from build123d import *

# Parameters (mm, degrees)
BOSS_EXTRUDE1_DEPTH = 152.4
SKETCH2_R           = 9.525
CUT_EXTRUDE1_DEPTH  = 187.6511184
CIRPATTERN1_COUNT   = 9
CIRPATTERN1_ANGLE   = 240


with BuildPart() as part:
    # Sketch1 → Boss-Extrude1 (new body)
    with BuildSketch(Plane.XY):
        with BuildLine():
            Line((0, 76.2), (0, 0))
            Line((0, 0), (76.2, 0))
            ThreePointArc((76.2, 0), (-53.881536726, -53.881536726), (0, 76.2))
        make_face()
    extrude(amount=-BOSS_EXTRUDE1_DEPTH)

    # Sketch2 → Cut-Extrude1 (cut, through all)
    with BuildSketch(Plane.XY):
        with Locations((-13.969757959, 52.135846474)):
            Circle(SKETCH2_R)
    cut_extrude1 = extrude(amount=-CUT_EXTRUDE1_DEPTH, mode=Mode.SUBTRACT)

    # CirPattern1: Cut-Extrude1 ×9 about axis, 1 skipped
    cirpattern1_axis = Axis((0, 0, 0), (0, 0, 1))
    add([cut_extrude1.rotate(cirpattern1_axis, i * CIRPATTERN1_ANGLE / (CIRPATTERN1_COUNT - 1)) for i in range(1, CIRPATTERN1_COUNT) if i not in (3,)], mode=Mode.SUBTRACT)


solid = part.part
The listing builds one solid part. Answer for the finished solid, in the listing's coordinates (mm). A direction names the side the tool comes from. Round coordinates to 2 decimals unless told otherwise and drop trailing zeros. Order: outer loops, then holes, each group sorted by start corner. A loop starts at its lowest first (then second) coordinate and runs counter-clockwise, first axis right, second up. Notation, with made-up numbers: M -31,77.25 L 11,77.25 A18 ccw 11,83.25 Z; hole C -19,2 d1. An arc over 180 degrees is marked long. Answer in a Markdown table with one row per item. Add a question column.
1) Which of the six approach directions +Z, -Z, +X, -X, +Y, -Y give full straight-line access (tool end or side, diameter ignored) to faces 5 (the face through (-16, -16, -152.4)), 6 (the face through (0, 39, -75))?
2) Flat-ended cylindrical pins translate along their axes: pin 1 Ø12 at (y, z) = (23, -68) entering from -X; pin 2 Ø1 at (x, y) = (46, -48.5) entering from +Z; pin 3 Ø2 at (x, z) = (2.5, -24) entering from +Y; pin 4 Ø12 at (y, z) = (-22.5, -134) entering from -X. Find the tip coordinate at first contact, or state that the pin passes through.
3) The part is cut by section C-C on z = -35. Count the separate pieces of the cut face and the enclosed holes in it, plus the area to 3 significant figures.
4) Consider line 1 along X through (y, z) = (-49, -89); line 2 along Y through (x, z) = (-37.5, -88); line 3 along Y through (x, z) = (-21.5, -99). Determine where each line is inside the solid, lowest interval first. Write a range as from..to.
5) Determine the mould class of faces 1 (the face through (-29.367, -41.814, -75.133)), 2 (the face through (-52.075, -55.629, -75.133)), 3 (the face through (-13.55, -42.62, -75.13)), 4 (the face through (38, 0, -75)) for opening direction X: pulls with the +X half, pulls with the -X half, needs draft (parallel to the pull), parting line crosses it, or undercut.
6) The part is cut by section D-D on y = 13.5. Determine the outline of the cut face in (x, z).
7) The part is cut by section A-A on y = 34.5. Determine the outline of the cut face in (x, z).
8) The part is cut by section B-B on x = -12. Determine the outline of the cut face in (y, z), plus the area to 3 significant figures.
Findings below:
| question | item | result |
|---|---|---|
| 1 | face 5 | -Z, +X, -X, +Y, -Y |
| 1 | face 6 | +Z, -Z, +X, +Y |
| 2 | pin 1 | stops at x = -74.28 |
| 2 | pin 2 | stops at z = 0 |
| 2 | pin 3 | stops at y = 0 |
| 2 | pin 4 | stops at x = -74.39 |
| 3 | separate pieces | 1 |
| 3 | enclosed holes | 8 |
| 3 | area | 11,400 mm² |
| 4 | line 1 | x = -58.36..-22.96, -4.98..4.98, 22.96..58.36 |
| 4 | line 2 | y = -66.33..-47.67, -28.66..28.66, 47.67..66.33 |
| 4 | line 3 | y = -73.1..-57.97, -46.3..46.3, 57.97..73.1 |
| 5 | face 1 | undercut |
| 5 | face 2 | parting line crosses it |
| 5 | face 3 | undercut |
| 5 | face 4 | needs draft |
| 6 | outline | M -74.99,-152.4 L -61.65,-152.4 L -61.65,0 L -74.99,0 Z; M -42.62,-152.4 L 0,-152.4 L 0,0 L -42.62,0 Z |
| 7 | outline | M -67.94,-152.4 L -46.96,-152.4 L -46.96,0 L -67.94,0 Z; M -29.37,-152.4 L 0,-152.4 L 0,0 L -29.37,0 Z |
| 8 | outline | M -75.25,-152.4 L -61.45,-152.4 L -61.45,0 L -75.25,0 Z; M -42.82,-152.4 L 42.82,-152.4 L 42.82,0 L -42.82,0 Z; M 61.45,-152.4 L 75.25,-152.4 L 75.25,0 L 61.45,0 Z |
| 8 | area | 17,300 mm² |
